The listing builds one solid part. Answer for the finished solid, in the listing's coordinates (mm). A direction names the side the tool comes from. Round coordinates to 2 decimals unless told otherwise and drop trailing zeros. Order: outer loops, then holes, each group sorted by start corner. A loop starts at its lowest first (then second) coordinate and runs counter-clockwise, first axis right, second up. Notation, with made-up numbers: (74, 54) - (89, 54) arc R34 cw to (89, 85) - close; hole circle Ø1 at (-37, -4). An arc over 180 degrees is marked (long way). One line per item, written item: value. Start each with the question number.
1. Flat-ended cylindrical pins translate along their axes: P1, Ø4, axis at x = 0.49, z = 192.5, coming from the -Y side; P2, Ø2.5, axis at y = 0.23, z = 177.5, coming from the -X side; P3, Ø6.5, axis at x = 0.49, z = 37.5, coming from the +Y side. Find the tip coordinate at first contact, or state that the pin passes through.
2. Straight lines are drawn through the part: line 1 (X direction, y = -1.25, z = 71.5); line 2 (Y direction, x = -2.75, z = 139); line 3 (X direction, y = 6.6, z = 192.5). For each, find the intervals that lie inside material, in ascending order.
3. A tool of negligible diameter and unlimited length cuts with its end or side. For faces 4 (the flat face through (0, 6.233, 99)), 5 (the cylindrical face through (-0.031, 6.993, 33.534)), 6 (the flat face through (0, 7.733, 99)), from which of +Z, -Z, +X, -X, +Y, -Y can it reach the whole face along a straight path? Write none if from no direction.
4. For a pull along Z with two mould halves and no side action, classify faces 1 (the flat face through (-6, 0, 200)), 2 (the flat face through (0, -5.767, 99)), 3 (the cylindrical face through (-0.4, -6.5, 3.6)) as released by +Z, released by -Z, zero draft, split by the parting line, or undercut.
5. Section A-A, the plane z = 80.5 is taken. Give the vertices of the cut face in (x, y).
6. Section B-B, the plane y = 3.5 is taken. Give the vertices of the cut face in (x, z), then the cut area to 3 significant figures.
from build123d import *

# Parameters (mm, degrees)
SKETCH_1_W          = 15
SKETCH_1_H          = 15
SKETCH_1_W_2        = 12
SKETCH_1_H_2        = 12
EXTRUDE_2_DEPTH     = 200
SKETCH_2_R          = 1.5
CUT_EXTRUDE_1_DEPTH = 15
SKETCH_3_R          = 1.5
CUT_EXTRUDE_2_DEPTH = 15
SKETCH_4_R          = 1.5
SKETCH_4_R_2        = 4
CUT_EXTRUDE_6_DEPTH = 10
SKETCH_6_R          = 1.5
SKETCH_6_R_2        = 4
CUT_EXTRUDE_7_DEPTH = 10


with BuildPart() as part:
    # ｽｹｯﾁ1 → ﾎﾞｽ - 押し出し2 (new body)
    with BuildSketch(Plane.XY):
        with Locations((0.489915859, 0.232626086)):
            Rectangle(SKETCH_1_W, SKETCH_1_H)
        with Locations((0.489915859, 0.232626086)):
            Rectangle(SKETCH_1_W_2, SKETCH_1_H_2, mode=Mode.SUBTRACT)
    extrude(amount=EXTRUDE_2_DEPTH)

    # ｽｹｯﾁ2 → ｶｯﾄ - 押し出し1 (cut)
    with BuildSketch(Plane(origin=(0, 7.732626086, 0), x_dir=(1, 0, 0), z_dir=(0, 1, 0))):
        with Locations((0.489915859, -192.5)):
            Circle(SKETCH_2_R)
    extrude(amount=-CUT_EXTRUDE_1_DEPTH, mode=Mode.SUBTRACT)

    # ｽｹｯﾁ3 → ｶｯﾄ - 押し出し2 (cut)
    with BuildSketch(Plane(origin=(7.989915859, 0, 0), x_dir=(0, 0, -1), z_dir=(1, 0, 0))):
        with Locations((-177.5, 0.232626086)):
            Circle(SKETCH_3_R)
    extrude(amount=-CUT_EXTRUDE_2_DEPTH, mode=Mode.SUBTRACT)

    # ｽｹｯﾁ4 → ｶｯﾄ - 押し出し6 (cut)
    with BuildSketch(Plane(origin=(0, 7.732626086, 0), x_dir=(1, 0, 0), z_dir=(0, 1, 0))):
        with Locations((0.489915859, -7.5)):
            Circle(SKETCH_4_R)
        with Locations((0.489915859, -37.5)):
            Circle(SKETCH_4_R_2)
    extrude(amount=-CUT_EXTRUDE_6_DEPTH, mode=Mode.SUBTRACT)

    # ｽｹｯﾁ6 → ｶｯﾄ - 押し出し7 (cut)
    with BuildSketch(Plane.XZ.offset(7.267373914)):
        with Locations((0.489915859, 37.5)):
            Circle(SKETCH_6_R)
        with Locations((0.489915859, 7.5)):
            Circle(SKETCH_6_R_2)
    extrude(amount=-CUT_EXTRUDE_7_DEPTH, mode=Mode.SUBTRACT)


solid = part.part
Answer list:
1. P1: stops at y = -7.27
1. P2: passes through
1. P3: stops at y = -5.77
2. line 1: x = -7.01 to -5.51, 6.49 to 7.99
2. line 2: y = -7.27 to -5.77, 6.23 to 7.73
2. line 3: x = -7.01 to -1.01, 1.99 to 7.99
3. face 4: +Z, -Z
3. face 5: +Y
3. face 6: +Z, -Z, +X, -X, +Y
4. face 1: released by +Z
4. face 2: zero draft
4. face 3: undercut
5. outline: (-7.01, -7.27) - (7.99, -7.27) - (7.99, 7.73) - (-7.01, 7.73) - close; hole (-5.51, -5.77) - (6.49, -5.77) - (6.49, 6.23) - (-5.51, 6.23) - close
6. outline: (-7.01, 0) - (-5.51, 0) - (-5.51, 200) - (-7.01, 200) - close; (6.49, 0) - (7.99, 0) - (7.99, 200) - (6.49, 200) - close
6. area: 600 mm²
